```python
from build123d import *

# Parameters (mm, degrees)
PAD_DEPTH              = 180
FUSION_PLACEMENT_ANGLE = 90
BOX_W                  = 46
BOX_H                  = 18
BOX_DEPTH              = 180
FILLET_R               = 5


with BuildPart() as pad:
    # Sketch → Pad (new body)
    with BuildSketch(Plane.XY):
        with BuildLine():
            Line((-4.01, 0), (-12.01, 0))
            Line((-12.01, 0), (-12.01, -6.353146))
            Line((-12.01, -6.353146), (-17, -11.343146))
            Line((-17, -11.343146), (-20, -11.343146))
            Line((-20, -11.343146), (-20, -5))
            Line((-20, -5), (-25, -5))
            Line((-25, -5), (-25, -20))
            ThreePointArc((-25, -20), (-23.535534, -23.535534), (-20, -25))
            Line((-20, -25), (-5, -25))
            Line((-5, -25), (-5, -20))
            Line((-5, -20), (-11.343146, -20))
            Line((-11.343146, -20), (-11.343146, -17))
            Line((-11.343146, -17), (-6.353146, -12.01))
            Line((-6.353146, -12.01), (0, -12.01))
            Line((0, -12.01), (0, -4.01))
            ThreePointArc((-4.01, 0), (-2.835498, -2.835498), (0, -4.01))
        make_face()
    extrude(amount=PAD_DEPTH)


with BuildPart() as part_mirroring:
    # Part__Mirroring: instance of Pad
    add(pad.part.mirror(Plane(origin=(0, 0, 0), x_dir=(1, 0, 0), z_dir=(0, 1, 0))))


with BuildPart() as fusion:
    # Fusion base: copy of Pad
    add(pad.part)

    # Fusion: union Part__Mirroring
    add(part_mirroring.part)


with BuildPart() as fusion_1:
    # Fusion placement: moved
    add(fusion.part.moved(Location((23, 25, 0))).rotate(Axis((23, 25, 0), (0, 0, 1)), FUSION_PLACEMENT_ANGLE))


with BuildPart() as fillet_body:
    # Box → Box (new body)
    with BuildSketch(Plane(origin=(0, -5, 0), x_dir=(1, 0, 0), z_dir=(0, 0, 1))):
        with Locations((23, 9)):
            Rectangle(BOX_W, BOX_H)
    extrude(amount=BOX_DEPTH)

    # Cut: cut Fusion
    add(fusion_1.part, mode=Mode.SUBTRACT)

    # Fillet
    fillet_edges = [fillet_body.edges().sort_by_distance(p)[0] for p in [
        (0, -5, 90),
        (46, -5, 90),
    ]]
    fillet(fillet_edges, radius=FILLET_R)


solid = fillet_body.part
```
Part model, mm, in its own coordinate system. A direction names the side the tool comes from. Give positions to 0.01 mm unless a question says otherwise; leave off trailing zeros. Loops run counter-clockwise (first coordinate to the right, second up) from the corner with the lowest first, then second, coordinate; pieces in that order, holes last. Notation, with made-up numbers: M -27,49 L -2,49 A24 cw -2,64 Z; hole C 76.5,-24.5 d2. An arc over 180 degrees is marked long. Return JSON: item names as keys, results as strings.
1) Saw through at B-B, the plane y = -3. List the corners of the cut face in (x, z).
Calculated:
{"outline": "M 1,0 L 45,0 L 45,180 L 1,180 Z"}
2) Flat gauge pins, fed straight in: pin 1 Ø7.5 at (x, z) = (10.5, 56) entering from +Y; pin 2 Ø3 at (x, z) = (39, 133) entering from +Y; pin 3 Ø2.5 at (y, z) = (6, 129.5) entering from +X. Where does each tip first touch, or does it go through?
Calculated:
{"pin 1": "stops at y = 10.59", "pin 2": "stops at y = 0", "pin 3": "stops at x = 34.34"}
3) 3-axis set-ups, long thin cutter, end or side, ignore diameter. For faces 4 (the face through (34.343, 7, 89)), 5 (the face through (15, 5, 89)), 6 (the face through (28, 3, 89)): which of +Z, -Z, +X, -X, +Y, -Y reach the whole face in a straight line?
Calculated:
{"face 4": "+Z, -Z, +X, +Y", "face 5": "+Z, -Z, -X", "face 6": "+Z, -Z"}
4) Saw through at C-C, the plane y = 9.5. List the corners of the cut face in (x, z), then the cut area to 3 significant figures.
Calculated:
{"outline": "M 13.16,0 L 32.84,0 L 32.84,180 L 13.16,180 Z", "area": "3,540 mm2"}
5) Pull direction Y, two halves, no side cores. Call faces 1 (the face through (31, 5, 89)), 2 (the face through (11.657, 7, 89)), 3 (the face through (44, -4, 91)): released by +Y, released by -Y, zero draft, split by the parting line, or undercut.
Calculated:
{"face 1": "undercut", "face 2": "zero draft", "face 3": "released by -Y"}
6) Saw through at A-A, the plane z = 63. List the corners of the cut face in (x, y).
Calculated:
{"outline": "M 0,0 A5 ccw 5,-5 L 41,-5 A5 ccw 46,0 L 46,1 A5 cw 43,0 L 28,0 L 28,5 L 34.34,5 L 34.34,8 L 29.35,12.99 L 16.65,12.99 L 11.66,8 L 11.66,5 L 18,5 L 18,0 L 3,0 A5 cw 0,1 Z"}
7) Drill centre lines: line 1 (X direction, y = 8, z = 7.5); line 2 (Y direction, x = 11, z = 138); line 3 (X direction, y = 0.5, z = 126.5). Where is each one in solid material? Low to high.
Calculated:
{"line 1": "x = 11.66 to 34.34", "line 2": "y = -5 to 0", "line 3": "x = 0 to 0.82, 18 to 28, 45.18 to 46"}
